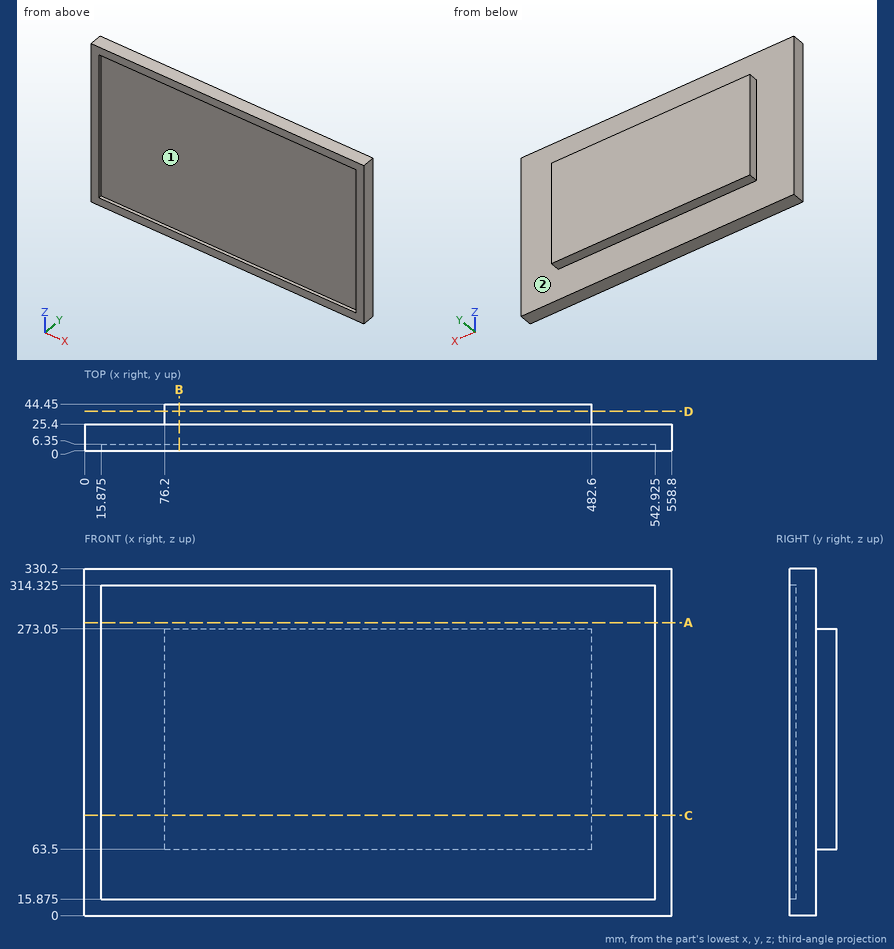
Geometry check sheet. Reference: drawing and pictorial views, mm from the part's lowest x, y, z. Round coordinates to 2 decimals unless told otherwise and drop trailing zeros. Order: outer loops, then holes, each group sorted by start corner. A loop starts at its lowest first (then second) coordinate and runs counter-clockwise, first axis right, second up. Notation, with made-up numbers: M 16,-36.75 L 68,-36.75 A32 cw 68,-2.75 Z; hole C -37,21.25 d7. An arc over 180 degrees is marked long. One line per item, written item: value. Start each with the question number.
1. Gauge pin test, flat ends, axial feed: P1, Ø5.5, axis at y = 36.5, z = 140.5, coming from the +X side; P2, Ø5.5, axis at x = 291.5, y = 31, coming from the -Z side; P3, Ø9.5, axis at y = 38.5, z = 177.5, coming from the -X side. Record the tip position at first contact, or that the pin passes through.
2. Section check A-A on z = 279. Enter the section's corners in (x, y) (3 decimals), and give its area (3 significant figures).
3. Section check D-D on y = 37.5. Enter the section's corners in (x, z).
4. Release check for a two-part mould opening along Z. For the marked faces 1 and 2 record: released by +Z, released by -Z, zero draft, split by the parting line, or undercut.
5. Section check C-C on z = 95.5. Enter the section's corners in (x, y) (3 decimals).
6. Section check B-B on x = 90. Enter the section's corners in (y, z) (3 decimals), and give its area (3 significant figures).
7. Scan lines: line 1 along Z through (x, y) = (26, 3) (3 decimals); line 2 along Y through (x, z) = (141, 297); line 3 along X through (y, z) = (39, 263). Record each from-to range of solid material in increasing order.
Results found:
1. P1: x = 482.6
1. P2: z = 63.5
1. P3: x = 76.2
2. outline: M 0,0 L 15.875,0 L 15.875,6.35 L 542.925,6.35 L 542.925,0 L 558.8,0 L 558.8,25.4 L 0,25.4 Z
2. area: 10,800 mm^2
3. outline: M 76.2,63.5 L 482.6,63.5 L 482.6,273.05 L 76.2,273.05 Z
4. face 1: undercut
4. face 2: zero draft
5. outline: M 0,0 L 15.875,0 L 15.875,6.35 L 542.925,6.35 L 542.925,0 L 558.8,0 L 558.8,25.4 L 482.6,25.4 L 482.6,44.45 L 76.2,44.45 L 76.2,25.4 L 0,25.4 Z
6. outline: M 0,0 L 25.4,0 L 25.4,63.5 L 44.45,63.5 L 44.45,273.05 L 25.4,273.05 L 25.4,330.2 L 0,330.2 L 0,314.325 L 6.35,314.325 L 6.35,15.875 L 0,15.875 Z
6. area: 10,500 mm^2
7. line 1: 0 to 15.875, 314.325 to 330.2
7. line 2: 6.35 to 25.4
7. line 3: 76.2 to 482.6
